CAD build for the part. Positions are in the model's coordinates, mm. Face numbers are marked on the shaded views. Round coordinates to 2 decimals unless told otherwise and drop trailing zeros. Order: outer loops, then holes, each group sorted by start corner. A loop starts at its lowest first (then second) coordinate and runs counter-clockwise, first axis right, second up.
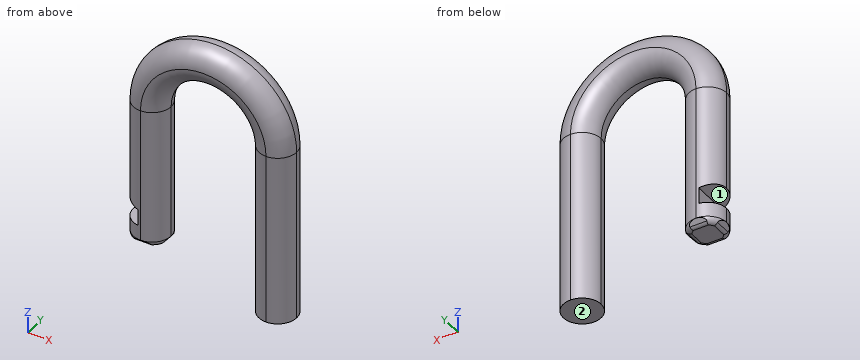
```python
from build123d import *

# Parameters (mm, degrees)
F0_W         = 7
F0_H         = 1
F1_DEPTH     = 7
F2_SIZE      = 1
F3_T1_DEPTH  = 40.75
F3_T3_DEPTH  = 33.75
F3_T5_DEPTH  = 27.1711544693
F3_T8_ANGLE  = 180
F3_T10_ANGLE = 180
F3_T12_ANGLE = 180
F3_T14_ANGLE = 180
F4_R         = 0.99999


# Not quite as in the source:
# - a fillet or chamfer that OpenCascade refuses, or shapes differently, is made with other operations: its cross-section is extruded or revolved along the edge and cut away or added
# - a fillet or chamfer is up to 0.001 mm smaller than in the source, because OpenCascade refuses the exact size


with BuildPart() as f1:
    # F0 (on Front) → F1 (new body)
    with BuildSketch(Plane.XZ):
        with BuildLine():
            ThreePointArc((-8.115, 0), (0, 8.115), (8.115, 0))
            Line((8.115, 0), (8.115, -32))
            Line((8.115, -32), (15.115, -32))
            Line((15.115, -32), (15.115, 0))
            ThreePointArc((15.115, 0), (0, 15.115), (-15.115, 0))
            Line((-15.115, 0), (-15.115, -18.4211544693))
            Line((-15.115, -18.4211544693), (-12.115, -19.3215445876))
            Line((-12.115, -19.3215445876), (-12.115, -22.3215445876))
            Line((-12.115, -22.3215445876), (-15.115, -22.3215445876))
            Line((-15.115, -22.3215445876), (-15.115, -25))
            Line((-15.115, -25), (-8.115, -25))
            Line((-8.115, -25), (-8.115, 0))
        make_face()
        with Locations((-11.615, -25.5)):
            Rectangle(F0_W, F0_H)
    extrude(amount=-F1_DEPTH)

    # F2
    f2_edges = [f1.edges().sort_by_distance(p)[0] for p in [
        (-8.115, 3.5, -26),
        (-11.615, 0, -26),
        (-11.615, 7, -26),
        (-15.115, 3.5, -26),
    ]]
    chamfer(f2_edges, length=F2_SIZE)

    # F3: fillet of radius 3.5 on 4 edges, made by hand

    # F3_s2 → F3_t1 (cut)
    with BuildSketch(Plane.XY.offset(-40.75)):
        with BuildLine():
            ThreePointArc((11.615, 0), (9.1401262658, 1.0251262658), (8.115, 3.5))
            Line((8.115, 3.5), (8.115, 0))
            Line((8.115, 0), (11.615, 0))
        make_face()
        with BuildLine():
            ThreePointArc((11.615, 0), (14.0898737342, 1.0251262658), (15.115, 3.5))
            Line((15.115, 3.5), (15.115, 0))
            Line((15.115, 0), (11.615, 0))
        make_face()
        with BuildLine():
            ThreePointArc((11.615, 7), (14.0898737342, 5.9748737342), (15.115, 3.5))
            Line((15.115, 3.5), (15.115, 7))
            Line((15.115, 7), (11.615, 7))
        make_face()
        with BuildLine():
            ThreePointArc((11.615, 7), (9.1401262658, 5.9748737342), (8.115, 3.5))
            Line((8.115, 3.5), (8.115, 7))
            Line((8.115, 7), (11.615, 7))
        make_face()
    extrude(amount=F3_T1_DEPTH, mode=Mode.SUBTRACT)

    # F3_s4 → F3_t3 (cut)
    with BuildSketch(Plane.XY.offset(-33.75)):
        with BuildLine():
            ThreePointArc((-11.615, 7), (-9.1401262658, 5.9748737342), (-8.115, 3.5))
            Line((-8.115, 3.5), (-8.115, 7))
            Line((-8.115, 7), (-11.615, 7))
        make_face()
        with BuildLine():
            ThreePointArc((-11.615, 0), (-9.1401262658, 1.0251262658), (-8.115, 3.5))
            Line((-8.115, 3.5), (-8.115, 0))
            Line((-8.115, 0), (-11.615, 0))
        make_face()
    extrude(amount=F3_T3_DEPTH, mode=Mode.SUBTRACT)

    # F3_s6 → F3_t5 (cut)
    with BuildSketch(Plane.XY.offset(-27.1711544693)):
        with BuildLine():
            ThreePointArc((-11.615, 7), (-14.0898737342, 5.9748737342), (-15.115, 3.5))
            Line((-15.115, 3.5), (-15.115, 7))
            Line((-15.115, 7), (-11.615, 7))
        make_face()
        with BuildLine():
            ThreePointArc((-11.615, 0), (-14.0898737342, 1.0251262658), (-15.115, 3.5))
            Line((-15.115, 3.5), (-15.115, 0))
            Line((-15.115, 0), (-11.615, 0))
        make_face()
    extrude(amount=F3_T5_DEPTH, mode=Mode.SUBTRACT)

    # F3_s7 → F3_t8 (revolve, cut)
    with BuildSketch(Plane.XY):
        with BuildLine():
            ThreePointArc((-11.615, 7), (-9.1401262658, 5.9748737342), (-8.115, 3.5))
            Line((-8.115, 3.5), (-8.115, 7))
            Line((-8.115, 7), (-11.615, 7))
        make_face()
    revolve(axis=Axis((0, 7, 0), (0, 1, 0)), revolution_arc=F3_T8_ANGLE, mode=Mode.SUBTRACT)

    # F3_s9 → F3_t10 (revolve, cut)
    with BuildSketch(Plane.XY):
        with BuildLine():
            ThreePointArc((11.615, 7), (14.0898737342, 5.9748737342), (15.115, 3.5))
            Line((15.115, 3.5), (15.115, 7))
            Line((15.115, 7), (11.615, 7))
        make_face()
    revolve(axis=Axis((0, 7, 0), (0, -1, 0)), revolution_arc=F3_T10_ANGLE, mode=Mode.SUBTRACT)

    # F3_s11 → F3_t12 (revolve, cut)
    with BuildSketch(Plane.XY):
        with BuildLine():
            ThreePointArc((11.615, 0), (14.0898737342, 1.0251262658), (15.115, 3.5))
            Line((15.115, 3.5), (15.115, 0))
            Line((15.115, 0), (11.615, 0))
        make_face()
    revolve(axis=Axis((0, 0, 0), (0, -1, 0)), revolution_arc=F3_T12_ANGLE, mode=Mode.SUBTRACT)

    # F3_s13 → F3_t14 (revolve, cut)
    with BuildSketch(Plane.XY):
        with BuildLine():
            ThreePointArc((-11.615, 0), (-9.1401262658, 1.0251262658), (-8.115, 3.5))
            Line((-8.115, 3.5), (-8.115, 0))
            Line((-8.115, 0), (-11.615, 0))
        make_face()
    revolve(axis=Axis((0, 0, 0), (0, 1, 0)), revolution_arc=F3_T14_ANGLE, mode=Mode.SUBTRACT)

    # F4 (radius 1 in the source; OpenCascade refuses exactly that, so slightly less here)
    f4_edges = [f1.edges().sort_by_distance(p)[0] for p in [
        (-11.615, 6, -26),
        (-14.115, 3.5, -26),
        (-11.615, 1, -26),
        (-9.115, 3.5, -26),
        (-9.140126, 5.974874, -26),
        (-14.089874, 5.974874, -26),
        (-14.089874, 1.025126, -26),
        (-9.140126, 1.025126, -26),
    ]]
    fillet(f4_edges, radius=F4_R)


solid = f1.part
```
1. Pin check, flat tips, straight feed: P1, Ø1, axis at x = 1, y = 2.5, coming from the -Z side; P2, Ø2, axis at x = 8, y = 1, coming from the +Z side; P3, Ø4, axis at x = -10.5, y = 4, coming from the -Z side. Stop position of each tip, or through.
2. Cut at B-B, the plane z = -28. Write the cut outline in (x, y) (3 decimals).
3. Drill centre lines: line 1 (X direction, y = 3.5, z = -25) (3 decimals); line 2 (X direction, y = 6, z = -16.5); line 3 (Y direction, x = 9.5, z = 0.5). Where is each one in solid material? Low to high.
4. Mould opens along Z. For the marked faces 1 and 2 say: released by +Z, released by -Z, zero draft, split by the parting line, or undercut.
5. Cut at A-A, the plane z = -9. Write the cut outline in (x, y) (3 decimals).
Outcome:
1. P1: stops at z = 8.06
1. P2: stops at z = 12.67
1. P3: stops at z = -26
2. outline: circle Ø7 at (11.615, 3.5)
3. line 1: x = -15.115 to -8.115, 8.115 to 15.115
3. line 2: x = -14.06 to -9.17, 9.17 to 14.06
3. line 3: y = 0.7 to 6.3
4. face 1: undercut
4. face 2: released by -Z
5. outline: circle Ø7 at (-11.615, 3.5); circle Ø7 at (11.615, 3.5)
